Geometry check sheet. Reference: the model listing, model coordinates, mm. Face numbers are marked on the shaded views. A direction names the side the tool comes from. Give positions to 0.01 mm unless a question says otherwise; leave off trailing zeros. Loops run counter-clockwise (first coordinate to the right, second up) from the corner with the lowest first, then second, coordinate; pieces in that order, holes last. Notation, with made-up numbers: (38, 59.5) -> (60, 59.5) arc R26 ccw to (60, 73.5) -> close; hole circle Ø10 at (5.5, 6.5). An arc over 180 degrees is marked (long way). One line per question, with ' | ' between items.
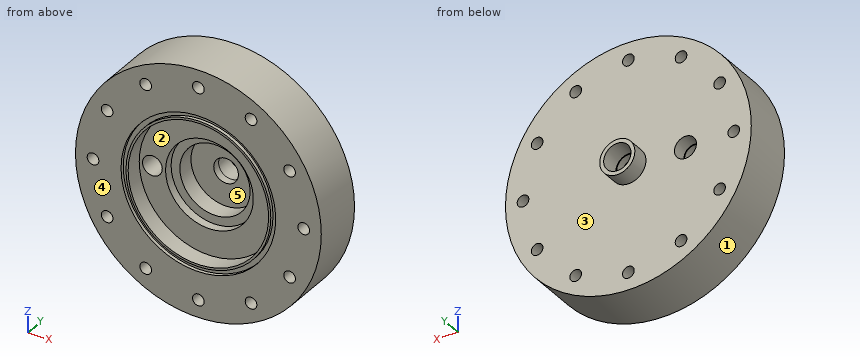
from build123d import *

# Parameters (mm, degrees)
F_5_16_CLEARANCE_HOLE1_D = 8.4328
CIRPATTERN1_COUNT        = 12


with BuildPart() as part:
    # Sketch1 → Revolve1 (revolve)
    with BuildSketch(Plane.XY):
        Polygon((-55.9435, 0), (-88.9, 0), (-88.9, 38.1), (-12.7, 38.1), (-12.7, 50.8), (0, 50.8), (0, 31.75), (-25.4, 31.75), (-25.4, 19.05), (-31.75, 19.05), (-31.75, 12.7), (-50.8, 12.7), (-50.8, 0), (-52.3875, 0), (-52.3875, 2.54), (-55.9435, 2.54), align=None)
    revolve(axis=Axis((0, 0, 0), (0, 1, 0)))

    # Sketch8 → 1/2 NPT Tapped Hole1 (revolve, cut)
    with BuildSketch(Plane(origin=(0, 50.8, 0), x_dir=(0, 0, 1), z_dir=(1, 0, 0))):
        Polygon((0, 0), (0, 50.8), (8.9281, 50.8), (8.9281, 13.462), (9.479726792, 13.462), (9.8827971, 0), align=None)
    revolve(axis=Axis((0, 57.15, 0), (0, -1, 0)), mode=Mode.SUBTRACT)

    # Sketch3 → 3/8 NPT Tapped Hole1 (revolve, cut)
    with BuildSketch(Plane(origin=(-41.275, 38.1, 0), x_dir=(0, 0, 1), z_dir=(1, 0, 0))):
        Polygon((0, 0), (0, 29.688582582), (7.1374, 25.4), (7.1374, 10.414), (7.653732494, 10.414), (7.9655416, 0), align=None)
    revolve(axis=Axis((-41.275, 44.45, 0), (0, -1, 0)), mode=Mode.SUBTRACT)

    # 5/16 Clearance Hole1 (through all)
    with Locations(Plane(origin=(0, 38.1, 0), x_dir=(1, 0, 0), z_dir=(0, 1, 0))):
        with Locations((-76.2, 0)):
            f_5_16_clearance_hole1 = Hole(F_5_16_CLEARANCE_HOLE1_D / 2)

    # CirPattern1: 5/16 Clearance Hole1 ×12 about axis
    cirpattern1_axis = Axis((0, 0, 0), (0, 1, 0))
    for i in range(1, CIRPATTERN1_COUNT):
        add(f_5_16_clearance_hole1.rotate(cirpattern1_axis, i * 360 / CIRPATTERN1_COUNT), mode=Mode.SUBTRACT)


solid = part.part
Item 1: Depth check by flat-ended pin: pin 1 Ø6 at (x, z) = (-12, -11) entering from +Y; pin 2 Ø7.5 at (x, z) = (38.1, 65.99) entering from +Y; pin 3 Ø1.5 at (x, y) = (-68.5, 17) entering from +Z; pin 4 Ø12 at (x, y) = (55.5, 20.5) entering from +Z. Enter the tip coordinate at first touch or a pass-through.
Result:
pin 1: y = 38.1 | pin 2: through | pin 3: z = 57.56 | pin 4: z = 73.84
Item 2: Release check for a two-part mould opening along Z. For the marked faces 1, 2 and 3 record: pulls with the +Z half, pulls with the -Z half, needs draft (parallel to the pull), parting line crosses it, or undercut.
Result:
face 1: parting line crosses it | face 2: undercut | face 3: needs draft
Item 3: Sectioned sample at B-B (x = 76.2). Record the cut outline in (y, z).
Result:
outline: (0, -45.79) -> (38.1, -45.79) -> (38.1, -4.22) -> (0, -4.22) -> close; (0, 4.22) -> (38.1, 4.22) -> (38.1, 45.79) -> (0, 45.79) -> close
Item 4: Sectioned sample at C-C (z = -76.2). Record the cut outline in (x, y).
Result:
outline: (-45.79, 0) -> (-4.22, 0) -> (-4.22, 38.1) -> (-45.79, 38.1) -> close; (4.22, 0) -> (45.79, 0) -> (45.79, 38.1) -> (4.22, 38.1) -> close
Item 5: Scan lines: probe 1 along X at (y, z) = (15, 5.5); probe 2 along Z at (x, y) = (38.1, 22); probe 3 along Y at (x, z) = (77, -7). Record each from-to range of solid material in increasing order.
Result:
probe 1: -88.73 to -45.82, -36.73 to -31.27, 31.27 to 88.73 | probe 2: -80.32 to -70.21, -61.77 to 61.77, 70.21 to 80.32 | probe 3: 0 to 38.1
Item 6: Sectioned sample at A-A (z = -38.1). Record the cut outline in (x, y).
Result:
outline: (-80.32, 0) -> (-70.21, 0) -> (-70.21, 38.1) -> (-80.32, 38.1) -> close; (-61.77, 0) -> (-40.96, 0) -> (-40.96, 2.54) -> (-35.96, 2.54) -> (-35.96, 0) -> (-33.6, 0) -> (-33.6, 12.7) -> (33.6, 12.7) -> (33.6, 0) -> (35.96, 0) -> (35.96, 2.54) -> (40.96, 2.54) -> (40.96, 0) -> (61.77, 0) -> (61.77, 38.1) -> (-61.77, 38.1) -> close; (70.21, 0) -> (80.32, 0) -> (80.32, 38.1) -> (70.21, 38.1) -> close
Item 7: Set-up check for the marked faces 4 and 5: record each of +Z, -Z, +X, -X, +Y, -Y from which the full face is reachable in a straight line by a thin tool's end or side.
Result:
face 4: +Z, -Z, +X, -X, -Y | face 5: -Y
Item 8: Sectioned sample at D-D (x = 19). Record the cut outline in (y, z), plus the area to 3 significant figures.
Result:
outline: (0, -86.85) -> (38.1, -86.85) -> (38.1, 86.85) -> (0, 86.85) -> (0, 52.62) -> (2.54, 52.62) -> (2.54, 48.82) -> (0, 48.82) -> (0, 47.11) -> (12.7, 47.11) -> (12.7, 25.44) -> (19.05, 25.44) -> (19.05, 16.86) -> (31.75, 16.86) -> (31.75, -16.86) -> (19.05, -16.86) -> (19.05, -25.44) -> (12.7, -25.44) -> (12.7, -47.11) -> (0, -47.11) -> (0, -48.82) -> (2.54, -48.82) -> (2.54, -52.62) -> (0, -52.62) -> close | area: 4,650 mm2
